Read the model definition and answer for the solid it produces. Units are mm, in the model's axes. Face numbers are marked on the shaded views. A direction names the side the tool comes from. Give positions to 0.01 mm unless a question says otherwise; leave off trailing zeros. Loops run counter-clockwise (first coordinate to the right, second up) from the corner with the lowest first, then second, coordinate; pieces in that order, holes last. Notation, with made-up numbers: (7, -28.5) - (31, -28.5) arc R6 ccw to (31, -22.5) - close; hole circle Ø9 at (-8.5, 54). An arc over 180 degrees is marked (long way). Write each question's results on one line, items separated by ' | '. Start each with the question number.
Q1. For the marked faces 1 and 2, determine the directions among +Z, -Z, +X, -X, +Y, -Y from which every point of the face is accessible in a straight line to the end or side of a thin tool.
Q2. The part is cut by section D-D, the plane z = -32. Write down the section's boundary in (x, y).
Q3. The part is cut by section C-C, the plane y = -9. Write down the section's boundary in (x, z).
Q4. The part is cut by section B-B, the plane x = 36. Write down the section's boundary in (y, z), plus the area to 3 significant figures.
Q5. Find the intervals of material crossed by line 1 (Y direction, x = 78.75, z = 2.15); line 2 (Y direction, x = 22.25, z = 0.8); line 3 (Y direction, x = 19, z = -3), in increasing order. Write a range as from..to.
Q6. Determine the mould class of the marked faces 3, 4 and 5 for opening direction X: +X half, -X half, draft (parallel to the pull), parting line (faces both ways), or undercut.
Q7. Given pin 1 (5 mm diameter, centred on x = 31, y = -1, fed in from -Z); pin 2 (5 mm diameter, centred on x = 116.75, y = -19.05, fed in from +Z), each flat-ended and moving along its own axis, determine where each tip first touches the part or whether it passes through.
Q8. The part is cut by section A-A, the plane x = 0. Write down the section's boundary in (y, z).
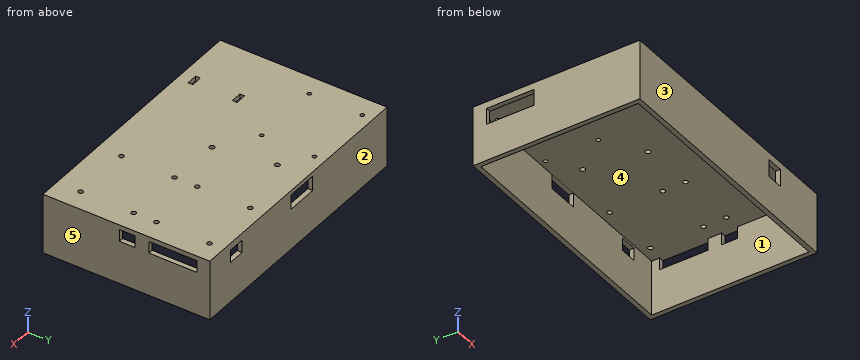
Autodesk Inventor part; units mm, degrees
ref_plane "YZ Plane" through (0, 0, 0) normal (1, 0, 0) x (0, 1, 0)
ref_plane "XZ Plane" through (0, 0, 0) normal (0, 1, 0) x (-1, 0, 0)
ref_plane "XY Plane" through (0, 0, 0) normal (0, 0, 1) x (1, 0, 0)
sketch "Эскиз1" plane through (0, 0, 0) normal (0, 0, 1) x (1, 0, 0)
  circle A0 centre (-22.25, 16.75) radius 1.25
  circle A1 centre (22.25, 16.75) radius 1.25
  circle A2 centre (22.25, -16.75) radius 1.25
  circle A3 centre (-22.25, -16.75) radius 1.25
  circle A4 centre (39.25, 4.75) radius 1.6
  circle A5 centre (45.54, -32.2859) radius 1.6
  circle A6 centre (78.75, -19.05) radius 1.5
  circle A7 centre (78.75, 14.55) radius 1.5
  circle A8 centre (116.75, 14.55) radius 1.5
  circle A9 centre (116.75, -19.05) radius 1.5
  circle A10 centre (116.75, -33.45) radius 1.5
  circle A11 centre (78.75, -33.45) radius 1.5
  circle A12 centre (78.75, -67.05) radius 1.5
  circle A13 centre (116.75, -67.05) radius 1.5
  line L0 (-19.75, -46.75) -> (24.25, -46.75)
  line L1 (24.25, -71.75) -> (-19.75, -71.75)
  line L2 (-1.6455, -46.75) -> (5.3545, -46.75)
  line L3 (5.3545, -46.75) -> (5.3545, -43.75)
  line L4 (5.3545, -43.75) -> (-1.6455, -43.75)
  line L5 (-1.6455, -43.75) -> (-1.6455, -46.75)
  line L6 (-1.6455, -71.75) -> (5.3545, -71.75)
  line L7 (5.3545, -71.75) -> (5.3545, -74.75)
  line L8 (5.3545, -74.75) -> (-1.6455, -74.75)
  line L9 (-1.6455, -74.75) -> (-1.6455, -71.75)
  line L10 (-32.25, 20.55) -> (126.75, 20.55)
  line L11 (126.75, 20.55) -> (126.75, -79.05)
  line L12 (126.75, -79.05) -> (-32.25, -79.05)
  line L13 (-32.25, -79.05) -> (-32.25, 20.55)
  point P0 (0, 0)
  dimension "d0" = 7
  dimension "d1" = 3
  dimension "d2" = 3
  dimension "d3" = 6
  dimension "d4" = 10
  dimension "d5" = 12
  dimension "d6" = 10
extrude "Выдавливание1" add sketch "Эскиз1" along normal blind 3
sketch "Эскиз2" plane through (0, 0, 0) normal (0, 0, -1) x (-1, 0, 0)
  line L0 (32.25, 20.55) -> (32.25, -79.05)
  line L1 (-126.75, -79.05) -> (-126.75, 20.55)
  line L2 (32.25, 20.55) -> (-126.75, 20.55)
  line L3 (-126.75, 20.55) -> (-126.75, -79.05)
  line L4 (-126.75, -79.05) -> (32.25, -79.05)
  line L5 (32.25, -79.05) -> (32.25, 20.55)
  line L6 (35.25, 23.55) -> (-129.75, 23.55)
  line L7 (-129.75, 23.55) -> (-129.75, -82.05)
  line L8 (-129.75, -82.05) -> (35.25, -82.05)
  line L9 (35.25, -82.05) -> (35.25, 23.55)
  point P0 (0, 0)
  point P1 (-126.75, 20.55)
  dimension "d9" = 3
  dimension "d10" = 3
  dimension "d11" = 3
  dimension "d12" = 3
extrude "Выдавливание2" add sketch "Эскиз2" along normal blind 35
sketch "Эскиз3" plane through (0, 0, 0) normal (0, 0, 1) x (1, 0, 0)
  line L0 (129.75, 23.55) -> (129.75, -82.05)
  line L1 (-35.25, 23.55) -> (129.75, 23.55)
  line L2 (-35.25, -82.05) -> (-35.25, 23.55)
  line L3 (129.75, -82.05) -> (-35.25, -82.05)
  line L4 (126.75, 20.55) -> (-32.25, 20.55)
  line L5 (126.75, -79.05) -> (126.75, 20.55)
  line L6 (-32.25, -79.05) -> (126.75, -79.05)
  line L7 (-32.25, 20.55) -> (-32.25, -79.05)
  point P0 (0, 0)
extrude "Выдавливание3" add sketch "Эскиз3" along normal blind 3
sketch "Эскиз4" plane through (-35.25, 23.55, -35) normal (0, 1, 0) x (1, 0, 0)
  line L0 (82.1894, -30.7775) -> (76.4292, -30.7775)
  line L1 (82.1894, -30.7775) -> (76.4292, -30.7775)
  line L2 (82.1894, -30.7775) -> (82.3893, -30.7775)
  line L3 (3, -35) -> (162, -35)
  line L4 (74.4292, -29.1972) -> (84.4292, -29.1972)
  line L5 (84.4292, -29.1972) -> (84.4292, -35)
  line L6 (84.4292, -35) -> (74.4292, -35)
  line L7 (74.4292, -35) -> (74.4292, -29.1972)
  point P0 (35.25, -35)
  dimension "d17" = 10
  dimension "d18" = 2
extrude "Выдавливание4" cut sketch "Эскиз4" against normal blind 3
sketch "Эскиз5" plane through (-35.25, 23.55, -35) normal (0, 1, 0) x (1, 0, 0)
  line L0 (74.4292, -35) -> (74.4292, -29.1972)
  line L1 (84.4292, -29.1972) -> (84.4292, -35)
  line L2 (74.4292, -29.1972) -> (84.4292, -29.1972)
  line L3 (84.4292, -35) -> (74.4292, -35)
  line L4 (69.2946, -35.2061) -> (89.2946, -35.2061)
  line L5 (89.2946, -35.2061) -> (89.2946, -25.902)
  line L6 (89.2946, -25.902) -> (69.2946, -25.902)
  line L7 (69.2946, -25.902) -> (69.2946, -35.2061)
  point P0 (35.25, -35)
  dimension "d21" = 20
extrude "Выдавливание5" cut sketch "Эскиз5" against normal blind 3
sketch "Эскиз6" plane through (-35.25, 23.55, -35) normal (0, 1, 0) x (1, 0, 0)
  line L0 (135, -33.5) -> (145.5, -33.5)
  line L1 (135, -33.5) -> (145.5, -33.5)
  line L2 (145.5, -25.5) -> (135, -25.5)
  line L3 (135, -33.5) -> (145.5, -33.5)
  line L4 (145.5, -33.5) -> (145.5, -25.5)
  line L5 (145.5, -25.5) -> (135, -25.5)
  line L6 (135, -25.5) -> (135, -33.5)
  point P0 (35.25, -35)
extrude "Выдавливание6" cut sketch "Эскиз6" against normal blind 3
sketch "Эскиз7" plane through (129.75, -82.05, -35) normal (1, 0, 0) x (0, 0, -1)
  line L0 (-27.42, 97.05) -> (-27.42, 67.05)
  line L1 (-35, 3) -> (-35, 102.6)
  line L2 (-35, 97.55) -> (-35, 100.05)
  line L3 (-27.42, 67.05) -> (-35, 67.05)
  line L4 (-35, 67.05) -> (-35, 97.55)
  line L5 (-35, 97.55) -> (-27.42, 97.55)
  line L6 (-27.42, 97.55) -> (-27.42, 67.05)
  line L7 (-33.5, 58.3) -> (-22.5, 58.3)
  line L8 (-35, 102.6) -> (-35, 3)
  line L9 (-27.42, 58.3) -> (-35, 58.3)
  line L10 (-35, 58.3) -> (-35, 48.4289)
  line L11 (-35, 48.4289) -> (-27.42, 48.4289)
  line L12 (-27.42, 48.4289) -> (-27.42, 58.3)
  point P0 (-35, 82.05)
  point P1 (-33.5, 58.3)
  point P2 (-35, 58.3)
  point P3 (-35, 48.4289)
  point P4 (-27.42, 97.05)
  point P5 (-35, 67.05)
extrude "Выдавливание7" cut sketch "Эскиз7" against normal blind 3
sketch "Эскиз8" plane through (-35.25, -82.05, -35) normal (0, -1, 0) x (1, 0, 0)
  line L0 (131, 33.5) -> (131, 22.5)
  line L1 (120.5, 33.5) -> (120.5, 22.5)
  line L2 (120.5, 22.5) -> (131, 22.5)
  line L3 (131, 22.5) -> (131, 33.5)
  line L4 (131, 33.5) -> (120.5, 33.5)
  line L5 (120.5, 33.5) -> (120.5, 22.5)
  point P0 (35.25, 35)
extrude "Выдавливание8" cut sketch "Эскиз8" against normal blind 3
sketch "Эскиз9" plane through (-35.25, -82.05, -35) normal (-1, 0, 0) x (0, 0, 1)
  line L0 (23.42, 97.05) -> (23.42, 67.05)
  line L1 (33.67, 64.8) -> (33.67, 99.3)
  line L2 (35, 67.05) -> (27.42, 67.05)
  line L3 (23.42, 97.05) -> (33.67, 97.05)
  line L4 (33.67, 97.05) -> (33.67, 67.05)
  line L5 (33.67, 67.05) -> (23.42, 67.05)
  line L6 (23.42, 67.05) -> (23.42, 97.05)
  point P0 (35, 82.05)
  point P1 (23.42, 67.05)
  point P2 (27.42, 67.05)
extrude "Выдавливание9" cut sketch "Эскиз9" against normal blind 3
properties part number "корпус"
Check sheet entries:
1) face 1: -Z | face 2: +Z, -Z, +X, -X, +Y
2) outline: (-35.25, -82.05) - (129.75, -82.05) - (129.75, 23.55) - (-35.25, 23.55) - close; hole (-32.25, -79.05) - (126.75, -79.05) - (126.75, 20.55) - (-32.25, 20.55) - close
3) outline: (-35.25, -35) - (-32.25, -35) - (-32.25, -11.58) - (-35.25, -11.58) - close; (-35.25, -1.33) - (-32.25, -1.33) - (-32.25, 0) - (129.75, 0) - (129.75, 3) - (-35.25, 3) - close; (126.75, -35) - (129.75, -35) - (129.75, -7.58) - (126.75, -7.58) - close
4) outline: (-82.05, -35) - (-79.05, -35) - (-79.05, 0) - (20.55, 0) - (20.55, 0.21) - (23.55, 0.21) - (23.55, 3) - (-82.05, 3) - close; (20.55, -35) - (23.55, -35) - (23.55, -9.1) - (20.55, -9.1) - close | area: 499 mm^2
5) line 1: y = -82.05..-68.55, -65.55..-34.95, -31.95..-20.55, -17.55..13.05, 16.05..23.55 | line 2: y = -82.05..-18, -15.5..15.5, 18..23.55 | line 3: y = -82.05..-79.05, 20.55..23.55
6) face 3: draft | face 4: undercut | face 5: +X half
7) pin 1: stops at z = 0 | pin 2: stops at z = 3
8) outline: (-82.05, -35) - (-79.05, -35) - (-79.05, 0) - (-74.75, 0) - (-74.75, 3) - (-82.05, 3) - close; (-71.75, 0) - (-46.75, 0) - (-46.75, 3) - (-71.75, 3) - close; (-43.75, 0) - (20.55, 0) - (20.55, -35) - (23.55, -35) - (23.55, 3) - (-43.75, 3) - close
